from build123d import *

# Parameters (mm, degrees)
BOSS_EXTRUDE1_DEPTH = 2
BOSS_EXTRUDE1_TAPER = 15
FILLET1_R           = 1
BOSS_EXTRUDE2_DEPTH = 3
BOSS_EXTRUDE2_DRAFT = 25
FILLET2_R           = 1
SKETCH4_W           = 26.928933456
SKETCH4_H           = 3.399397771
BOSS_EXTRUDE3_DEPTH = 3
BOSS_EXTRUDE3_TAPER = 10
FILLET3_START       = 3.548118457
FILLET3_DEPTH       = 3.399397771


with BuildPart() as part:
    # Sketch2 → Boss-Extrude1 (new body)
    with BuildSketch(Plane(origin=(0, 0, 0), x_dir=(1, 0, 0), z_dir=(0, 1, 0))):
        Polygon((2.245194627, -15.051216937), (4.446052988, 10.654239994), (-3.553947012, 10.654239994), (-1.754805373, -15.051216937), align=None)
    extrude(amount=BOSS_EXTRUDE1_DEPTH, taper=BOSS_EXTRUDE1_TAPER)

    # Fillet1
    fillet1_edges = [part.edges().sort_by_distance(p)[0] for p in [
        (2.807764808, 2, 2.198488472),
        (0.441540754, 2, -10.118341609),
        (-2.117166811, 2, 2.198488472),
        (0.249057243, 2, 14.515318552),
    ]]
    fillet(fillet1_edges, radius=FILLET1_R)


with BuildPart() as boss_extrude2_tool:
    # Sketch3 → Boss-Extrude2 (with draft: the straight prism first)
    with BuildSketch(Plane(origin=(0, 0, 0), x_dir=(1, 0, 0), z_dir=(0, 1, 0))):
        with BuildLine():
            Line((-12.679718033, 5.755185759), (14.192118481, 5.755185759))
            ThreePointArc((14.192118481, 5.755185759), (0.756200224, 15.248268586), (-12.679718033, 5.755185759))
        make_face()
    extrude(amount=BOSS_EXTRUDE2_DEPTH)
    # Boss-Extrude2: the draft: its side faces are tilted about the plane it starts from
    boss_extrude2_sides = [boss_extrude2_tool.faces().sort_by_distance(p)[0] for p in [
        (0.756200224, 1.5, -5.755185759),
        (0.756200224, 1.5, -15.248268586),
    ]]
    draft(boss_extrude2_sides, Plane(origin=(0, 0, 0), x_dir=(1, 0, 0), z_dir=(0, 1, 0)), BOSS_EXTRUDE2_DRAFT)


with BuildPart() as part_1:
    add(part.part)

    # Boss-Extrude2: add boss_extrude2_tool
    add(boss_extrude2_tool.part)

    # Fillet2
    fillet2_edges = [part_1.edges().sort_by_distance(p)[0] for p in [
        (0.756200224, 3, -7.154108734),
        (0.756200224, 3, -13.849345612),
    ]]
    fillet(fillet2_edges, radius=FILLET2_R)

    # Sketch4 → Boss-Extrude3 (add)
    with BuildSketch(Plane(origin=(0, 0, 0), x_dir=(1, 0, 0), z_dir=(0, 1, 0))):
        with Locations((0, -5.247817343)):
            Rectangle(SKETCH4_W, SKETCH4_H)
    extrude(amount=BOSS_EXTRUDE3_DEPTH, taper=BOSS_EXTRUDE3_TAPER)

    # Fillet3: read off the stored shape, not the designer's step
    # Fillet3 outline → Fillet3 (cut)
    with BuildSketch(Plane.XY.offset(FILLET3_START)):
        with BuildLine():
            Line((12.935485786, 3), (7.371907057, 3))
            add(Edge.make_bspline(
                [(7.371907057, 3), (12.935485786, 3), (13.280753575, 1.041889066)],
                knots=[0, 0, 0, 1, 1, 1], degree=2, weights=[1, 0.766044443, 1]))
            Line((13.280753575, 1.041889066), (12.935485786, 3))
        make_face()
        with BuildLine():
            add(Edge.make_bspline(
                [(-7.371907057, 3), (-12.935485786, 3), (-13.280753575, 1.041889066)],
                knots=[0, 0, 0, 1, 1, 1], degree=2, weights=[1, 0.766044443, 1]))
            Line((-7.371907057, 3), (-12.935485786, 3))
            Line((-12.935485786, 3), (-13.280753575, 1.041889066))
        make_face()
    extrude(amount=FILLET3_DEPTH, mode=Mode.SUBTRACT)


solid = part_1.part
Verification items for the finished model (mm, model axes). A direction names the side the tool comes from. Round coordinates to 2 decimals unless told otherwise and drop trailing zeros. Answer in a Markdown table with one row per item. Add a question column.
Q1. Material ranges on line 1 (Z direction, x = -1.5, y = 2.25); line 2 (Z direction, x = -5.75, y = 2.45); line 3 (Y direction, x = -1.25, z = -1.5), recorded low to high.
Q2. Gauge pin test, flat ends, axial feed: pin 1 (5 mm diameter, centred on x = 0.5, z = -3.5, fed in from +Y); pin 2 (10 mm diameter, centred on x = 2, z = -2.5, fed in from -Y). Record the tip position at first contact, or that the pin passes through.
Q3. Tool access check on faces 5 (the face through (0, 2, 10)), 6 (the face through (1, 3, -10)), 7 (the face through (0.92, 2.84, -7.25)). Record the directions out of +Z, -Z, +X, -X, +Y, -Y that give a thin tool (end or side, any length) a straight path to the whole face; none if there is none.
Q4. Release check for a two-part mould opening along Z. For faces 1 (the face through (0, 2, -1)), 2 (the face through (0.568, 2.271, -6.814)), 3 (the face through (0, 3, 5)), 4 (the face through (0.98, 2.27, -14.19)) record: pulls with the +Z half, pulls with the -Z half, needs draft (parallel to the pull), parting line crosses it, or undercut.
Found:
| question | item | result |
|---|---|---|
| 1 | line 1 | z = -14 to -6.8, 3.94 to 6.55 |
| 1 | line 2 | z = -12.38 to -6.9, 3.98 to 6.52 |
| 1 | line 3 | y = 0 to 2 |
| 2 | pin 1 | stops at y = 2 |
| 2 | pin 2 | stops at y = 0 |
| 3 | face 5 | +Z, +X, -X, +Y |
| 3 | face 6 | +Z, -Z, +X, -X, +Y |
| 3 | face 7 | +X, -X, +Y |
| 4 | face 1 | undercut |
| 4 | face 2 | undercut |
| 4 | face 3 | needs draft |
| 4 | face 4 | pulls with the -Z half |
